Verification items for this drawing (mm, ordinates from the low corner). A direction names the side the tool comes from. Round coordinates to 2 decimals unless told otherwise and drop trailing zeros. Write each loop counter-clockwise with the first axis right and the second up, starting at its lowest first coordinate (ties: lowest second). Pieces come first, ordered by that corner, then holes.
Item 1: Access from +Z, -Z, +X, -X, +Y, -Y to the whole of each face (thin tool, end or side, straight path). Record for the marked faces 3, 4 and 5.
Item 2: Draft check along Z on the marked faces 1 and 2. Enter one of: pulls with the +Z half, pulls with the -Z half, needs draft (parallel to the pull), parting line crosses it, or undercut.
Item 3: Cross-section at C-C (x = 8). Enter the section's corners in (y, z), then the cut area to 3 significant figures.
Item 4: Cross-section at B-B (x = 24.13). Enter the section's corners in (y, z), then the cut area to 3 significant figures.
Item 5: Cross-section at A-A (y = 57.15). State how many separate pieces and enclosed holes the cut face has, then the cut area to 3 significant figures.
Item 6: Depth check by flat-ended pin: P1, Ø4.5, axis at y = 19.05, z = 28.575, coming from the +X side (3 decimals); P2, Ø1.5, axis at x = 19, y = 43, coming from the -Z side; P3, Ø10, axis at x = 59.5, z = 46.5, coming from the +Y side. Enter the tip coordinate at first touch or a pass-through.
Item 7: Scan lines: probe 1 along Z at (x, y) = (24.13, 38); probe 2 along Y at (x, z) = (42, 65). Record each from-to range of solid material in increasing order.
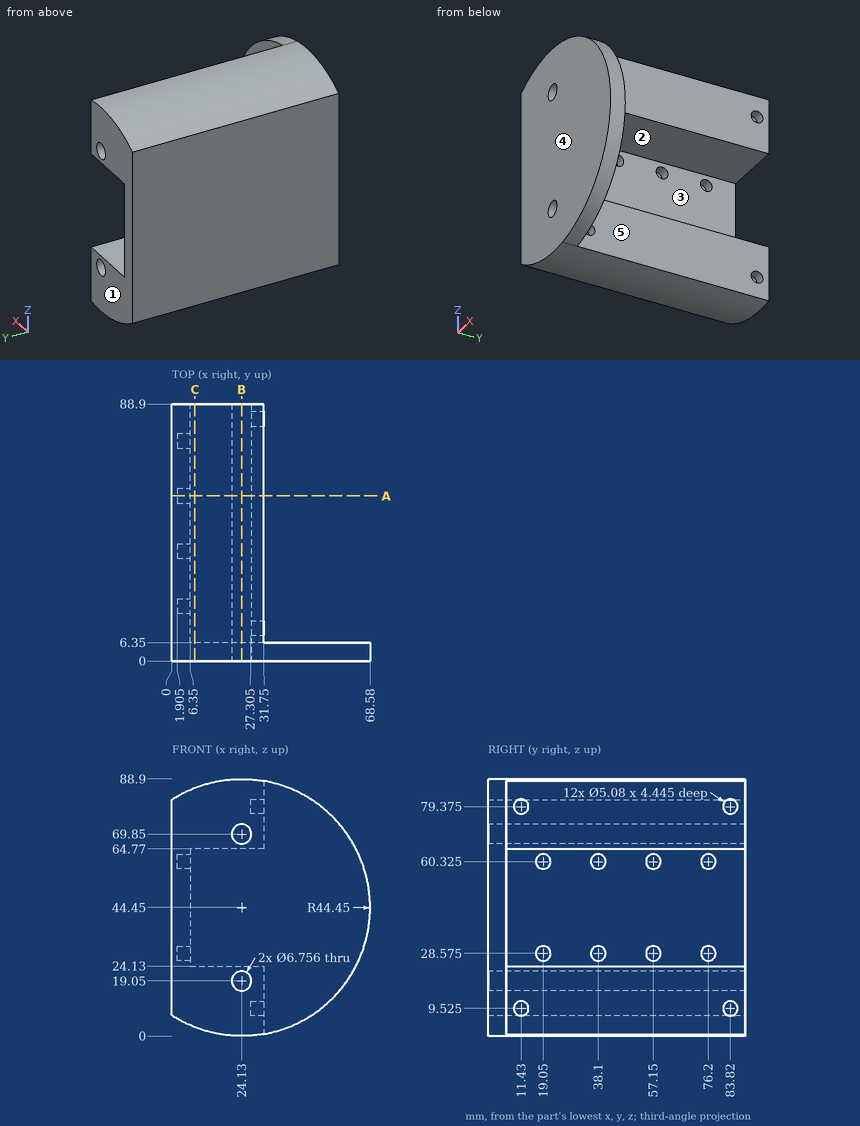
Resolved:
1. face 3: +X, +Y
1. face 4: +Z, -Z, +X, -X, -Y
1. face 5: +Z, -Z, +X, +Y
2. face 1: needs draft
2. face 2: undercut
3. outline: (0, 3.03) - (88.9, 3.03) - (88.9, 24.13) - (6.35, 24.13) - (6.35, 64.77) - (88.9, 64.77) - (88.9, 85.87) - (0, 85.87) - close
3. area: 4,010 mm2
4. outline: (0, 0) - (88.9, 0) - (88.9, 15.67) - (0, 15.67) - close; (0, 22.43) - (88.9, 22.43) - (88.9, 24.13) - (6.35, 24.13) - (6.35, 64.77) - (88.9, 64.77) - (88.9, 66.47) - (0, 66.47) - close; (0, 73.23) - (88.9, 73.23) - (88.9, 88.9) - (0, 88.9) - close
4. area: 3,350 mm2
5. separate pieces: 1
5. enclosed holes: 2
5. area: 1,560 mm2
6. P1: stops at x = 1.905
6. P2: stops at z = 0.22
6. P3: stops at y = 6.35
7. probe 1: z = 0 to 15.67, 22.43 to 24.13, 64.77 to 66.47, 73.23 to 88.9
7. probe 2: y = 0 to 6.35
